Could you check a few things on this model? Use its own coordinates, in mm. A direction names the side the tool comes from. Round coordinates to 2 decimals unless told otherwise and drop trailing zeros. Order: outer loops, then holes, each group sorted by start corner. A loop starts at its lowest first (then second) coordinate and runs counter-clockwise, first axis right, second up. Notation, with made-up numbers: (23.25, -25.5) - (80.25, -25.5) arc R16 cw to (80.25, -2.5) - close; hole circle Ø11 at (72, 32.5). An arc over 180 degrees is marked (long way). Use one line per item in the form item = value.
from build123d import *

# Parameters (mm, degrees)
BOSS_EXTRUDE1_DEPTH = 2
BOSS_EXTRUDE2_DEPTH = 10
BOSS_EXTRUDE3_DEPTH = 10
SKETCH3_R           = 1.6
CUT_EXTRUDE1_DEPTH  = 10
BOSS_EXTRUDE4_DEPTH = 1
MOVE_FACE1_DEPTH    = 10
BOSS_EXTRUDE5_DEPTH = 0.5


# Read off the part's stored shape, not the designer's step: Move Face1
with BuildPart() as part:
    # Sketch1 → Boss-Extrude1 (new body)
    with BuildSketch(Plane.XY):
        with BuildLine():
            Line((0, 17), (0, 1.65))
            ThreePointArc((0, 1.65), (-1.65, 0), (0, -1.65))
            Line((0, -1.65), (0, -17))
            ThreePointArc((0, -17), (-17, 0), (0, 17))
        make_face()
    extrude(amount=BOSS_EXTRUDE1_DEPTH)

    # Sketch2 → Boss-Extrude2 (add)
    with BuildSketch(Plane.XY):
        with BuildLine():
            Line((0, 17), (0, 18.5))
            ThreePointArc((0, 18.5), (-18.5, 0), (0, -18.5))
            Line((0, -18.5), (0, -17))
            ThreePointArc((0, -17), (-17, 0), (0, 17))
        make_face()
    extrude(amount=BOSS_EXTRUDE2_DEPTH)

    # Sketch4 → Boss-Extrude3 (add)
    with BuildSketch(Plane.XY.offset(10)):
        Polygon((0, -18.5), (-1.127101366, -17.373839009), (-2, -17.373839009), (-2, -22.499993139), (-2, -26.5), (0, -26.5), align=None)
    boss_extrude3 = extrude(amount=-BOSS_EXTRUDE3_DEPTH)

    # Sketch3 → Cut-Extrude1 (cut)
    with BuildSketch(Plane(origin=(0, 0, 0), x_dir=(0, 0, -1), z_dir=(1, 0, 0))):
        with Locations(Location((-5, -22.5, 0), (0, 0, 90))):
            Circle(SKETCH3_R)
    cut_extrude1 = extrude(amount=-CUT_EXTRUDE1_DEPTH, mode=Mode.SUBTRACT)

    # Sketch5 → Boss-Extrude4 (add)
    with BuildSketch(Plane(origin=(0, 0, 0), x_dir=(-1, 0, 0), z_dir=(0, 0, -1))):
        Polygon((2, -26.5), (6.889586723, -17.169263082), (2, -17.169263082), align=None)
    boss_extrude4 = extrude(amount=-BOSS_EXTRUDE4_DEPTH)

    # Mirror1: Boss-Extrude3, Cut-Extrude1, Boss-Extrude4 across plane
    add(boss_extrude3.mirror(Plane.ZX))
    add(cut_extrude1.mirror(Plane.ZX), mode=Mode.SUBTRACT)
    add(boss_extrude4.mirror(Plane.ZX))

    # Move Face1 outline → Move Face1 (cut)
    with BuildSketch(Plane.XY):
        with BuildLine():
            ThreePointArc((-0.1, 1.747140521), (-1.75, 0), (-0.1, -1.747140521))
            Line((-0.1, -1.747140521), (-0.1, -26.5))
            Line((-0.1, -26.5), (0, -26.5))
            Line((0, -26.5), (0, -1.65))
            ThreePointArc((0, -1.65), (-1.65, 0), (0, 1.65))
            Line((0, 1.65), (0, 26.5))
            Line((0, 26.5), (-0.1, 26.5))
            Line((-0.1, 26.5), (-0.1, 1.747140521))
        make_face()
    extrude(amount=MOVE_FACE1_DEPTH, mode=Mode.SUBTRACT)

    # Sketch6 → Boss-Extrude5 (add)
    with BuildSketch(Plane.XY.offset(2)):
        with BuildLine():
            Line((-0.1, 13.099618315), (-0.1, 12.09958677))
            ThreePointArc((-0.1, 12.09958677), (-12.1, 0), (-0.1, -12.09958677))
            Line((-0.1, -12.09958677), (-0.1, -13.099618315))
            ThreePointArc((-0.1, -13.099618315), (-13.1, 0), (-0.1, 13.099618315))
        make_face()
    extrude(amount=BOSS_EXTRUDE5_DEPTH)


solid = part.part
Item 1: Will these pins go through, and if not, where does the flat tip stop? P1, Ø1.5, axis at x = -5.5, y = 22.5, coming from the +Z side; P2, Ø10, axis at x = -4, y = -0.5, coming from the -Z side; P3, Ø2, axis at x = -7, z = 8, coming from the -Y side; P4, Ø1.5, axis at y = 10, z = 8, coming from the -X side.
Found:
P1 = through
P2 = 0
P3 = -17.5
P4 = -16.02
Item 2: Imagine slicing it at D-D on y = -22.5. Please give me the cut outline in (x, z).
Found:
outline = (-4.1, 0) - (-0.1, 0) - (-0.1, 3.4) - (-2, 3.4) - (-2, 1) - (-4.1, 1) - close; (-2, 6.6) - (-0.1, 6.6) - (-0.1, 10) - (-2, 10) - close
Item 3: Imagine slicing it at B-B on y = 0. Please give me the cut outline in (x, z), plus the area to 3 significant figures.
Found:
outline = (-18.5, 0) - (-1.75, 0) - (-1.75, 2) - (-12.1, 2) - (-12.1, 2.5) - (-13.1, 2.5) - (-13.1, 2) - (-17, 2) - (-17, 10) - (-18.5, 10) - close
area = 46.0 mm2
Item 4: If we mould it in two halves opening along Z, with no side actions, what happens to faces 1 (the face through (-12.3, 0.1, 2.5)), 2 (the face through (-1, 26.5, 5)), 3 (the face through (-1.04, 21.02, 4.39))? For each: released by +Z, released by -Z, zero draft, split by the parting line, or undercut.
Found:
face_1 = released by +Z
face_2 = zero draft
face_3 = undercut
Item 5: I need wall thicknesses on L1, parallel to Z at x = -0.8, y = -22.5; L2, parallel to X at y = 20, z = 1.5; L3, parallel to Z at x = -12.75, y = 1.5. Which ranges of each line are inside material? Lowest first, please.
Found:
L1 = 0 to 3.4, 6.6 to 10
L2 = -2 to -0.1
L3 = 0 to 2.5
Item 6: Imagine slicing it at C-C on x = -16.25. Please give me the cut outline in (y, z).
Found:
outline = (-8.84, 0) - (8.84, 0) - (8.84, 10) - (4.99, 10) - (4.99, 2) - (-4.99, 2) - (-4.99, 10) - (-8.84, 10) - close
Item 7: For faces 4 (the face through (-2, -23, 7)), 5 (the face through (-12.097, 0.265, 2.246)), 6 (the face through (-18.496, 0.379, 4.93)), which set-ups out of +Z, -Z, +X, -X, +Y, -Y let a thin tool reach every point of the face, with its end or its side?
Found:
face_4 = +Z, -X, -Y
face_5 = +Z, +X
face_6 = +Z, -X
